```python
from build123d import *

# Parameters (mm, degrees)
EXTRUDE_1_OUTLINE_W = 40
EXTRUDE_1_OUTLINE_H = 20
EXTRUDE_1_DEPTH     = 4
SKETCH_2_R          = 1.5
CUT_EXTRUDE_1_DEPTH = 47.69047012
SKETCH_3_W          = 7
SKETCH_3_H          = 2
CUT_EXTRUDE_2_DEPTH = 2
FILLET_1_R          = 1


# Read off the part's stored shape, not the designer's step: 凸台-拉伸1
with BuildPart() as part:
    # 凸台-拉伸1 outline → 凸台-拉伸1 (new body)
    with BuildSketch(Plane(origin=(0, 0, 0), x_dir=(1, 0, 0), z_dir=(0, 1, 0))):
        Polygon((-27, -15), (-5, -15), (-5, -20), (5, -20), (5, -15), (22, -15), (27, -20), (35, -20), (35, -12), (42, -5), (42, 5), (35, 12), (35, 20), (27, 20), (22, 15), (5, 15), (5, 20), (-5, 20), (-5, 15), (-27, 15), align=None)
        Rectangle(EXTRUDE_1_OUTLINE_W, EXTRUDE_1_OUTLINE_H, mode=Mode.SUBTRACT)
    extrude(amount=EXTRUDE_1_DEPTH)

    # 草图2 → 切除-拉伸1 (cut, through all)
    with BuildSketch(Plane(origin=(0, 4, 0), x_dir=(1, 0, 0), z_dir=(0, 1, 0))):
        with Locations(Location((0, 15, 0), (0, 0, 270))):
            Circle(SKETCH_2_R)
        with Locations(Location((0, -15, 0), (0, 0, 90))):
            Circle(SKETCH_2_R)
        with Locations(Location((29, 14, 0), (0, 0, 270))):
            Circle(SKETCH_2_R)
        with Locations(Location((29, -14, 0), (0, 0, 90))):
            Circle(SKETCH_2_R)
        with Locations(Location((37, 0, 0), (0, 0, 270))):
            Circle(SKETCH_2_R)
    extrude(amount=-CUT_EXTRUDE_1_DEPTH, mode=Mode.SUBTRACT)

    # 草图3 → 切除-拉伸2 (cut)
    with BuildSketch(Plane.XZ):
        with Locations((-23.5, 0)):
            Rectangle(SKETCH_3_W, SKETCH_3_H)
        with Locations((23.5, 0)):
            Rectangle(SKETCH_3_W, SKETCH_3_H)
    extrude(amount=-CUT_EXTRUDE_2_DEPTH, mode=Mode.SUBTRACT)

    # 圆角1
    fillet_1_edges = [part.edges().sort_by_distance(p)[0] for p in [
        (-27, 2, 15),
        (-27, 2, -15),
        (-5, 2, -15),
        (-5, 2, -20),
        (5, 2, -20),
        (5, 2, -15),
        (22, 2, -15),
        (27, 2, -20),
        (35, 2, -20),
        (35, 2, -12),
        (42, 2, -5),
        (42, 2, 5),
        (35, 2, 12),
        (35, 2, 20),
        (27, 2, 20),
        (22, 2, 15),
        (5, 2, 15),
        (5, 2, 20),
        (-5, 2, 20),
        (-5, 2, 15),
    ]]
    fillet(fillet_1_edges, radius=FILLET_1_R)


solid = part.part
```
Here's how the part is built. I have some questions about the finished solid (model axes, mm). A direction names the side the tool comes from. Give positions to 0.01 mm unless a question says otherwise; leave off trailing zeros. Order: outer loops, then holes, each group sorted by start corner. A loop starts at its lowest first (then second) coordinate and runs counter-clockwise, first axis right, second up. Notation, with made-up numbers: M 46,51.25 L 52,51.25 A22 ccw 52,87.25 Z; hole C 27.25,75.25 d7. An arc over 180 degrees is marked long. Use a Markdown table: item, result. Add a question column.
1. Suppose I cut it at B-B (z = -7). List the corners of the cut face in (x, y) for me, and give its area (3 significant figures).
2. On a 3-axis mill with a long thin cutter (end or side, diameter ignored), from which of +Z, -Z, +X, -X, +Y, -Y can I reach the whole of each face in a straight line? I mean faces 4 (the flat face through (27, 1, 0)), 5 (the flat face through (20, 2.4, 0.1)), 6 (the flat face through (-5, 2, -18)), 7 (the flat face through (24, 2, 17)). Say none if no direction works.
3. I need wall thicknesses on probe 1 along X at (y, z) = (2.8, 0); probe 2 along Z at (x, y) = (-16.5, 1.7); probe 3 along Z at (x, y) = (-3, 0.5). Which ranges of each line are inside material? Lowest first, please. Write a range as from..to.
4. Suppose I cut it at A-A (x = 29). List the corners of the cut face in (y, z) for me.
5. Suppose I cut it at D-D (z = -11). List the corners of the cut face in (x, y) for me, and give its area (3 significant figures).
6. For pin 1 Ø2 at (y, z) = (3.5, -13.5) entering from +X; pin 2 Ø1.5 at (y, z) = (3, -18) entering from -X; pin 3 Ø0.6 at (x, y) = (24.5, 1.5) entering from -Z, each with a flat end and sliding along its axis, tell me the tip position at first contact or that it passes through.
7. Suppose I cut it at C-C (x = -13). List the corners of the cut face in (y, z) for me.
8. If we mould it in two halves opening along Z, with no side actions, what happens to faces 1 (the flat face through (14, 2, -15)), 2 (the flat face through (38, 2, 9)), 3 (the cylindrical face through (27.99, 2.03, 15.11))? For each: +Z half, -Z half, draft (parallel to the pull), parting line (faces both ways), or undercut.
Results list:
| question | item | result |
|---|---|---|
| 1 | outline | M -27,0 L -20,0 L -20,4 L -27,4 Z; M 20,0 L 40,0 L 40,4 L 20,4 Z |
| 1 | area | 108 mm² |
| 2 | face 4 | -X, -Y |
| 2 | face 5 | +Y, -Y |
| 2 | face 6 | -Z, -X, +Y, -Y |
| 2 | face 7 | +Z, +Y, -Y |
| 3 | probe 1 | x = -27..-20, 20..35.5, 38.5..42 |
| 3 | probe 2 | z = -15..-10, 10..15 |
| 3 | probe 3 | z = -20..-10, 10..20 |
| 4 | outline | M 0,-20 L 4,-20 L 4,-15.5 L 0,-15.5 Z; M 0,-12.5 L 4,-12.5 L 4,12.5 L 0,12.5 Z; M 0,15.5 L 4,15.5 L 4,20 L 0,20 Z |
| 5 | outline | M -27,0 L 36,0 L 36,4 L -27,4 Z |
| 5 | area | 252 mm² |
| 6 | pin 1 | stops at x = 35 |
| 6 | pin 2 | stops at x = -5 |
| 6 | pin 3 | stops at z = -17.8 |
| 7 | outline | M 0,-15 L 4,-15 L 4,-10 L 0,-10 Z; M 0,10 L 4,10 L 4,15 L 0,15 Z |
| 8 | face 1 | -Z half |
| 8 | face 2 | +Z half |
| 8 | face 3 | undercut |
